Work out the finished part from the listing and answer in its coordinate system (mm). Coordinates: 2 decimals unless noted, no trailing zeros. Order: outer loops, then holes, each group sorted by start corner. A loop starts at its lowest first (then second) coordinate and runs counter-clockwise, first axis right, second up. Notation, with made-up numbers: (10, -40) -> (32, -40) arc R20 cw to (32, -10) -> close; hole circle Ø9 at (69, -23). An arc over 180 degrees is marked (long way). Write item = value, one per line. Start each with the question number.
Q1. The part is cut by section C-C, the plane y = -8. Determine the outline of the cut face in (x, z), plus the area to 3 significant figures.
Q2. The part is cut by section B-B, the plane x = 17. Determine the outline of the cut face in (y, z).
Q3. The part is cut by section A-A, the plane z = 0.7. Determine the outline of the cut face in (x, y), plus the area to 3 significant figures.
Q4. Straight lines are drawn through the part: L1, parallel to X at y = 25, z = 2; L2, parallel to X at y = -24.5, z = 1.5; L3, parallel to Y at x = 28.5, z = 0.45. For each, find the intervals that lie inside material, in ascending order. Write a range as from..to.
Q5. Flat-ended cylindrical pins translate along their axes: pin 1 (1.5 mm diameter, centred on x = 15.5, z = 1.5, fed in from -Y); pin 2 (1 mm diameter, centred on y = -14.5, z = 1.5, fed in from +X); pin 3 (1.5 mm diameter, centred on y = 25, z = 1.5, fed in from -X). Find the tip coordinate at first contact, or state that the pin passes through.
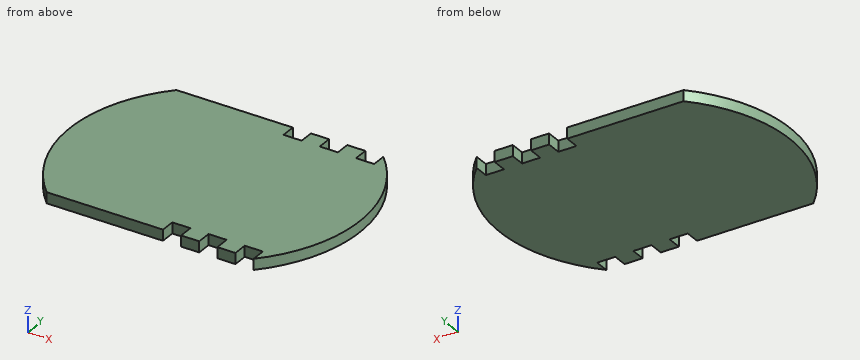
Autodesk Inventor part; units mm, degrees
ref_plane "YZ Plane" through (0, 0, 0) normal (1, 0, 0) x (0, 1, 0)
ref_plane "XZ Plane" through (0, 0, 0) normal (0, 1, 0) x (-1, 0, 0)
ref_plane "XY Plane" through (0, 0, 0) normal (0, 0, 1) x (1, 0, 0)
sketch "Sketch1" plane through (0, 0, 0) normal (0, 0, 1) x (1, 0, 0)
  line L0 (0, 28) -> (-28.5657, 28)
  line L1 (-42.7333, 0) -> (57.4636, 0) construction
  line L2 (0, -28) -> (-28.5657, -28)
  arc A0 (-28.5657, 28) -> (-28.5657, -28) centre (0, 0) ccw
  arc A1 (28.5657, -28) -> (28.5657, 28) centre (0, 0) ccw
  line L3 (28.5657, 28) -> (28.5657, 24)
  line L4 (28.5657, 24) -> (23.5657, 24)
  line L5 (23.5657, 24) -> (23.5657, 28)
  line L6 (23.5657, 28) -> (18.5657, 28)
  line L7 (18.5657, 28) -> (18.5657, 24)
  line L8 (18.5657, 24) -> (13.5657, 24)
  line L9 (13.5657, 24) -> (13.5657, 28)
  line L10 (13.5657, 28) -> (8.5657, 28)
  line L11 (8.5657, 28) -> (8.5657, 24)
  line L12 (8.5657, 24) -> (3.5657, 24)
  line L13 (3.5657, 24) -> (3.5657, 28)
  line L14 (0, 28) -> (3.5657, 28)
  line L15 (8.5657, 28) -> (13.5657, 28)
  line L16 (28.5657, -28) -> (28.5657, -24)
  line L17 (28.5657, -24) -> (23.5657, -24)
  line L18 (23.5657, -24) -> (23.5657, -28)
  line L19 (23.5657, -28) -> (18.5657, -28)
  line L20 (18.5657, -28) -> (18.5657, -24)
  line L21 (18.5657, -24) -> (13.5657, -24)
  line L22 (13.5657, -24) -> (13.5657, -28)
  line L23 (13.5657, -28) -> (8.5657, -28)
  line L24 (8.5657, -28) -> (8.5657, -24)
  line L25 (8.5657, -24) -> (3.5657, -24)
  line L26 (3.5657, -24) -> (3.5657, -28)
  line L27 (8.5657, -28) -> (13.5657, -28)
  line L28 (0, -28) -> (3.5657, -28)
  line L29 (8.5657, -28) -> (13.5657, -28)
  line L30 (18.5657, -28) -> (23.5657, -28)
  dimension "d2" = 40
  dimension "d3" = 40
  dimension "d4" = 4
  dimension "d9" = 5
  dimension "d17" = 4
  dimension "d18" = 4
  dimension "d20" = 4
  dimension "d21" = 4
extrude "Extrusion1" add sketch "Sketch1" along normal blind 3
equation "\"d3\" = d2"
equation "\"d17\" = d4"
equation "\"d18\" = d4"
equation "\"d20\" = d4"
equation "\"d21\" = d4"
properties part number "base"
Model answer:
q1.outline = (-39.19, 0) -> (39.19, 0) -> (39.19, 3) -> (-39.19, 3) -> close
q1.area = 235 mm2
q2.outline = (-24, 0) -> (24, 0) -> (24, 3) -> (-24, 3) -> close
q3.outline = (-28.57, -28) -> (3.57, -28) -> (3.57, -24) -> (8.57, -24) -> (8.57, -28) -> (13.57, -28) -> (13.57, -24) -> (18.57, -24) -> (18.57, -28) -> (23.57, -28) -> (23.57, -24) -> (28.57, -24) -> (28.57, -28) arc R40 ccw to (28.57, 28) -> (28.57, 24) -> (23.57, 24) -> (23.57, 28) -> (18.57, 28) -> (18.57, 24) -> (13.57, 24) -> (13.57, 28) -> (8.57, 28) -> (8.57, 24) -> (3.57, 24) -> (3.57, 28) -> (-28.57, 28) arc R40 ccw to start
q3.area = 3,960 mm2
q4.L1 = -31.22..3.57, 8.57..13.57, 18.57..23.57, 28.57..31.22
q4.L2 = -31.62..3.57, 8.57..13.57, 18.57..23.57, 28.57..31.62
q4.L3 = -24..24
q5.pin_1 = -24
q5.pin_2 = 37.47
q5.pin_3 = -31.81
